Work out the finished part from the listing and answer in its coordinate system (mm). Face numbers are marked on the shaded views. A direction names the side the tool comes from. Round coordinates to 2 decimals unless told otherwise and drop trailing zeros. Loops run counter-clockwise (first coordinate to the right, second up) from the corner with the lowest first, then second, coordinate; pieces in that order, holes last. Notation, with made-up numbers: (76.25, 31.5) - (114.25, 31.5) arc R25 cw to (114.25, 68.5) - close; hole circle Ø7 at (-6, -28). An arc over 180 degrees is marked (long way). Return JSON: item names as keys, results as strings.
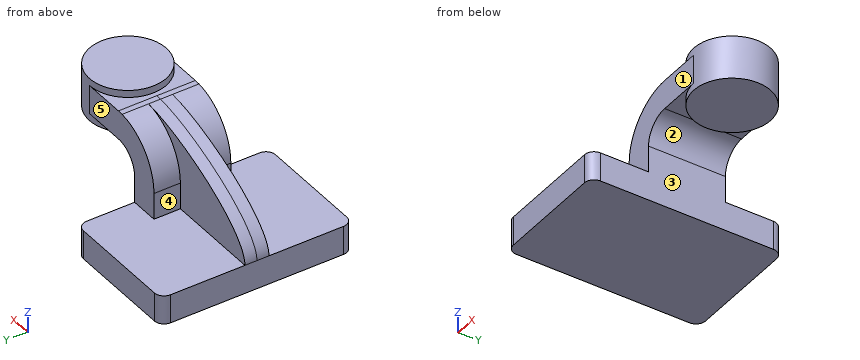
from build123d import *

# Parameters (mm, degrees)
F1_DEPTH = 63.5
F2_DEPTH = 25.4
F0_W     = 25.4
F0_H     = 19.05
F3_DEPTH = 25.4
F4_DEPTH = 7.9375
F6_R     = 6.35


with BuildPart() as f1:
    # F0 (on Front) → F1 (new body, symmetric)
    with BuildSketch(Plane.XZ):
        Polygon((-41.275, 9.525), (-41.275, -9.525), (41.275, -9.525), (41.275, 9.525), (22.225, 9.525), align=None)
    extrude(amount=F1_DEPTH, both=True)

    # F0 (on Front) → F2 (join, symmetric)
    with BuildSketch(Plane.XZ):
        with BuildLine():
            Line((22.225, 9.525), (41.275, 9.525))
            Line((41.275, 9.525), (41.275, 27.0002))
            ThreePointArc((41.275, 27.0002), (45.9246798487, 38.2255201513), (57.15, 42.8752))
            Line((57.15, 42.8752), (60.325, 42.8752))
            Line((60.325, 42.8752), (60.325, 61.9252))
            Line((60.325, 61.9252), (57.15, 61.9252))
            add(Edge.make_bspline(
                [(53.5742223952, 61.7416657077), (54.8066544525, 61.8373665684), (56.0001082359, 61.8990472552), (57.15, 61.9252)],
                knots=[107.5074121299, 107.5074121299, 107.5074121299, 107.5074121299, 111.5045361635, 111.5045361635, 111.5045361635, 111.5045361635], degree=3))
            ThreePointArc((53.5742223952, 61.7416657077), (31.2208691059, 50.3975459195), (22.225, 27.0002))
            Line((22.225, 27.0002), (22.225, 9.525))
        make_face()
    extrude(amount=F2_DEPTH, both=True)

    # F0 (on Front) → F3 (join, symmetric)
    with BuildSketch(Plane.XZ):
        with Locations((73.025, 52.4002)):
            Rectangle(F0_W, F0_H)
    extrude(amount=F3_DEPTH, both=True)

    # F0 (on Front) → F4 (join, symmetric)
    with BuildSketch(Plane.XZ):
        with BuildLine():
            add(Edge.make_bspline(
                [(-41.275, 9.525), (-40.9183161587, 31.9833210844), (20.4264941805, 59.1676770631), (53.5742223952, 61.7416657077)],
                knots=[0, 0, 0, 0, 107.5074121299, 107.5074121299, 107.5074121299, 107.5074121299], degree=3))
            Line((-41.275, 9.525), (22.225, 9.525))
            Line((22.225, 9.525), (22.225, 27.0002))
            ThreePointArc((22.225, 27.0002), (31.2208691059, 50.3975459195), (53.5742223952, 61.7416657077))
        make_face()
    extrude(amount=F4_DEPTH, both=True)

    # F0 (on Front) → F5 (revolve)
    with BuildSketch(Plane.XZ):
        Polygon((85.725, 66.675), (85.725, 61.9252), (85.725, 42.8752), (85.725, 38.1), (111.125, 38.1), (111.125, 66.675), align=None)
    revolve(axis=Axis((85.725, 0, 52.3875), (0, 0, 1)))

    # F6
    f6_edges = [f1.edges().sort_by_distance(p)[0] for p in [
        (-41.275, -63.5, 0),
        (41.275, -63.5, 0),
        (-41.275, 63.5, 0),
        (41.275, 63.5, 0),
    ]]
    fillet(f6_edges, radius=F6_R)


solid = f1.part
1) A tool of negligible diameter and unlimited length cuts with its end or side. For the marked faces 1, 2, 3, 4 and 5, from which of +Z, -Z, +X, -X, +Y, -Y can it reach the whole face along a straight path? Write none if from no direction.
Verdict:
{"face 1": "+Z, +X, -X, -Y", "face 2": "-Z, +Y, -Y", "face 3": "-Z, +X, +Y, -Y", "face 4": "+Z, -X, +Y", "face 5": "+Z, +X, -X, +Y"}
2) Flat-ended cylindrical pins translate along their axes: pin 1 (14 mm diameter, centred on y = -17.5, z = 21.5, fed in from -X) (3 decimals); pin 2 (5 mm diameter, centred on x = 72.5, y = 13, fed in from -Z); pin 3 (19 mm diameter, centred on y = 12.5, z = 16.5, fed in from -X) (3 decimals); pin 4 (2 mm diameter, centred on x = -21.5, y = 3, fed in from +Z). Find the tip coordinate at first contact, or state that the pin passes through.
Verdict:
{"pin 1": "stops at x = 22.225", "pin 2": "stops at z = 38.1", "pin 3": "stops at x = -41.275", "pin 4": "stops at z = 34.81"}
3) Section A-A (z = -2.5) is taken. Give the vertices of the cut face in (x, y) (3 decimals), and give its area (3 significant figures).
Verdict:
{"outline": "(-41.275, -57.15) arc R6.35 ccw to (-34.925, -63.5) - (34.925, -63.5) arc R6.35 ccw to (41.275, -57.15) - (41.275, 57.15) arc R6.35 ccw to (34.925, 63.5) - (-34.925, 63.5) arc R6.35 ccw to (-41.275, 57.15) - close", "area": "10,400 mm2"}
4) Section B-B (y = -43.5) is taken. Give the vertices of the cut face in (x, z) (3 decimals), and give its area (3 significant figures).
Verdict:
{"outline": "(-41.275, -9.525) - (41.275, -9.525) - (41.275, 9.525) - (-41.275, 9.525) - close", "area": "1,570 mm2"}
5) Find the intervals of material crossed by L1, parallel to X at y = 52.5, z = -3.5 (3 decimals); L2, parallel to Z at x = 4, y = 33 (3 decimals); L3, parallel to Y at x = 29, z = 12.5, in increasing order.
Verdict:
{"L1": "x = -41.275 to 41.275", "L2": "z = -9.525 to 9.525", "L3": "y = -25.4 to 25.4"}
